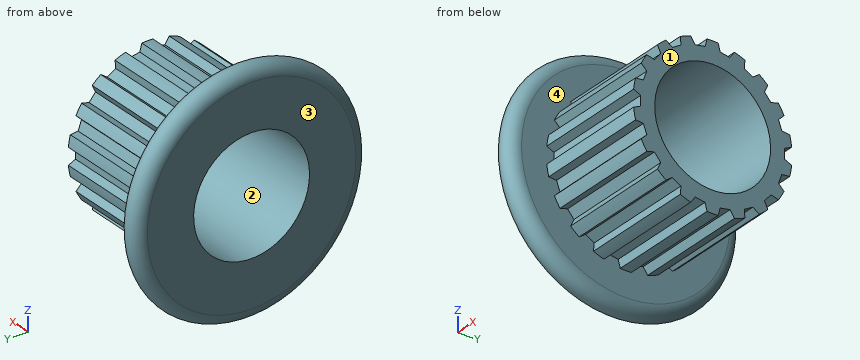
from build123d import *

# Parameters (mm, degrees)
SKETCH4_R          = 5.8
SKETCH4_R_2        = 5.4825
CUT_EXTRUDE2_DEPTH = 8
CUT_EXTRUDE1_DEPTH = 8
CIRPATTERN1_COUNT  = 18


with BuildPart() as part:
    # Sketch1 → Revolve1 (revolve)
    with BuildSketch(Plane.XY, mode=Mode.PRIVATE) as revolve1_sk:
        with BuildLine():
            Line((-1.6, 4), (8, 4))
            Line((8, 4), (8, 5.55))
            Line((8, 5.55), (0, 5.55))
            Line((0, 5.55), (0, 7.2))
            ThreePointArc((0, 7.2), (-0.8, 8), (-1.6, 7.2))
            Line((-1.6, 7.2), (-1.6, 4))
        make_face()
    revolve(revolve1_sk.sketch.rotate(Axis((-1.6, 0, 0), (1, 0, 0)), 90), axis=Axis((-1.6, 0, 0), (1, 0, 0)))

    # Sketch4 → Cut-Extrude2 (cut)
    with BuildSketch(Plane(origin=(0, 0, 0), x_dir=(0, 0, -1), z_dir=(1, 0, 0))):
        Circle(SKETCH4_R)
        with Locations(Location((0, 0, 0), (0, 0, 180))):
            Circle(SKETCH4_R_2, mode=Mode.SUBTRACT)
    extrude(amount=CUT_EXTRUDE2_DEPTH, mode=Mode.SUBTRACT)

    # Sketch3 → Cut-Extrude1 (cut)
    with BuildSketch(Plane(origin=(0, 0, 0), x_dir=(0, 0, -1), z_dir=(1, 0, 0))):
        with BuildLine():
            Line((-0.642345316, 5.604560113), (-0.343021997, 4.962659182))
            Line((-0.343021997, 4.962659182), (0.343021997, 4.962659182))
            Line((0.343021997, 4.962659182), (0.642345316, 5.604560113))
            ThreePointArc((0.642345316, 5.604560113), (0, 5.64125), (-0.642345316, 5.604560113))
        make_face()
    cut_extrude1 = extrude(amount=CUT_EXTRUDE1_DEPTH, mode=Mode.SUBTRACT)

    # CirPattern1: Cut-Extrude1 ×18 about axis
    cirpattern1_axis = Axis((0, 0, 0), (1, 0, 0))
    for i in range(1, CIRPATTERN1_COUNT):
        add(cut_extrude1.rotate(cirpattern1_axis, i * 360 / CIRPATTERN1_COUNT), mode=Mode.SUBTRACT)


solid = part.part
The listing builds one solid part. Answer for the finished solid, in the listing's coordinates (mm). Face numbers are marked on the shaded views. A direction names the side the tool comes from. Coordinates: 2 decimals unless noted, no trailing zeros. Loops run counter-clockwise (first coordinate to the right, second up) from the corner with the lowest first, then second, coordinate; pieces in that order, holes last. Notation, with made-up numbers: (-6, 5) -> (49, 5) arc R21 ccw to (49, 40) -> close; hole circle Ø4 at (22.25, 55.25). An arc over 180 degrees is marked (long way). Write item = value, one per line. Start each with the question number.
1) Given pin 1 Ø1.5 at (x, z) = (4, 2.5) entering from +Y, flat-ended and moving along its own axis, determine where the tip first touches the part or whether it passes through.
2) Straight lines are drawn through the part: line 1 (Y direction, x = 2, z = 0); line 2 (Y direction, x = 2.75, z = 1); line 3 (Z direction, x = 0.5, y = -1.75). For each, find the intervals that lie inside material, in ascending order. Write a range as from..to.
3) A tool of negligible diameter and unlimited length cuts with its end or side. For the marked faces 3 and 4, from which of +Z, -Z, +X, -X, +Y, -Y can it reach the whole face along a straight path? Write none if from no direction.
4) A cutting plane is placed at A-A (z = 0). Give the vertices of the cut face in (x, y), then the cut area to 3 significant figures.
5) The mould has two halves that part along Z. Classify the marked faces 1 and 2: released by +Z, released by -Z, zero draft, split by the parting line, or undercut.
6) A cutting plane is placed at B-B (y = 0). Give the vertices of the cut face in (x, z), then the cut area to 3 significant figures.
Responses:
q1.pin_1 = 4.93
q2.line_1 = -4.96..-4, 4..4.96
q2.line_2 = -5.39..-3.87, 3.87..5.39
q2.line_3 = -5.2..-3.6, 3.6..5.2
q3.face_3 = +Z, -Z, -X, +Y, -Y
q3.face_4 = +X
q4.outline = (-1.6, -7.2) arc R0.8 ccw to (0, -7.2) -> (0, -4.96) -> (8, -4.96) -> (8, -4) -> (-1.6, -4) -> close; (-1.6, 4) -> (8, 4) -> (8, 4.96) -> (0, 4.96) -> (0, 7.2) arc R0.8 ccw to (-1.6, 7.2) -> close
q4.area = 27.7 mm²
q5.face_1 = zero draft
q5.face_2 = undercut
q6.outline = (-1.6, -7.2) arc R0.8 ccw to (0, -7.2) -> (0, -5.48) -> (8, -5.48) -> (8, -4) -> (-1.6, -4) -> close; (-1.6, 4) -> (8, 4) -> (8, 5.48) -> (0, 5.48) -> (0, 7.2) arc R0.8 ccw to (-1.6, 7.2) -> close
q6.area = 36.0 mm²
